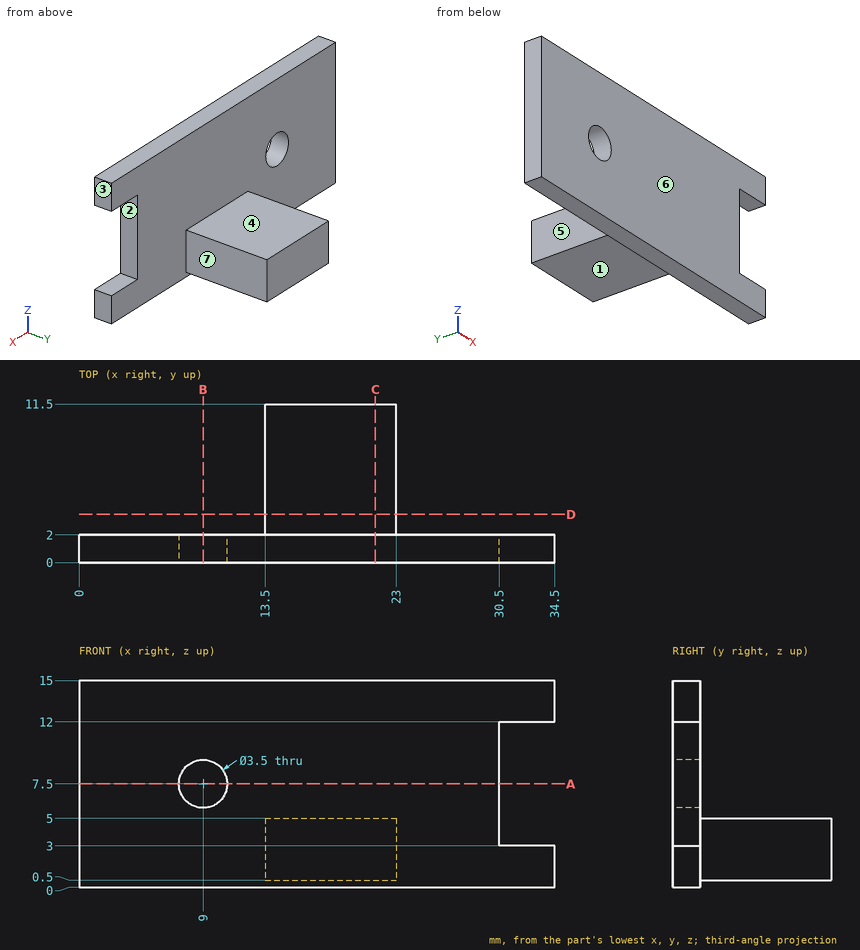
Geometry check sheet. Reference: drawing and pictorial views, mm from the part's lowest x, y, z. A direction names the side the tool comes from. Give positions to 0.01 mm unless a question says otherwise; leave off trailing zeros. Order: outer loops, then holes, each group sorted by start corner. A loop starts at its lowest first (then second) coordinate and runs counter-clockwise, first axis right, second up. Notation, with made-up numbers: M 36.25,1 L 43.25,1 A5 cw 43.25,5 Z; hole C 30.25,-10.5 d4. An arc over 180 degrees is marked long. Return JSON: item names as keys, results as strings. Group by question number.
1) Section check D-D on y = 3.5. Record the cut outline in (x, z).
2) Access from +Z, -Z, +X, -X, +Y, -Y to the whole of each face (thin tool, end or side, straight path). Record for the marked faces 4, 5, 6 and 7.
3) Go/stop test with flat-tipped pins: pin 1 Ø6 at (y, z) = (9.5, 5.5) entering from +X; pin 2 Ø5 at (y, z) = (5.5, 4) entering from -X; pin 3 Ø4.5 at (x, z) = (26, 8.5) entering from +Y. Record where each tip stops, or that it passes through.
4) Section check C-C on x = 21.5. Record the cut outline in (y, z), and give its area (4 significant figures).
5) Mould release check, pull along Z, two halves, no side actions. Record for the marked faces 1, 2 and 3: pulls with the +Z half, pulls with the -Z half, needs draft (parallel to the pull), parting line crosses it, or undercut.
6) Scan lines: line 1 (X direction, y = 0.4, z = 7.5); line 2 (Z direction, x = 9, y = 1.1); line 3 (Z direction, x = 15.5, y = 2.25). Record each from-to range of solid material in increasing order.
7) Section check B-B on x = 9. Record the cut outline in (y, z).
8) Section check A-A on z = 7.5. Record the cut outline in (x, y), and give its area (3 significant figures).
Answer block:
{
 "1": {"outline": "M 13.5,0.5 L 23,0.5 L 23,5 L 13.5,5 Z"},
 "2": {"face 4": "+Z, +X, -X, +Y", "face 5": "+Z, -Z, -X, +Y", "face 6": "+Z, -Z, +X, -X, -Y", "face 7": "+Z, -Z, +X, +Y"},
 "3": {"pin 1": "stops at x = 23", "pin 2": "stops at x = 13.5", "pin 3": "stops at y = 2"},
 "4": {"outline": "M 0,0 L 2,0 L 2,0.5 L 11.5,0.5 L 11.5,5 L 2,5 L 2,15 L 0,15 Z", "area": "72.75 mm^2"},
 "5": {"face 1": "pulls with the -Z half", "face 2": "undercut", "face 3": "needs draft"},
 "6": {"line 1": "x = 0 to 7.25, 10.75 to 30.5", "line 2": "z = 0 to 5.75, 9.25 to 15", "line 3": "z = 0.5 to 5"},
 "7": {"outline": "M 0,0 L 2,0 L 2,5.75 L 0,5.75 Z; M 0,9.25 L 2,9.25 L 2,15 L 0,15 Z"},
 "8": {"outline": "M 0,0 L 7.25,0 L 7.25,2 L 0,2 Z; M 10.75,0 L 30.5,0 L 30.5,2 L 10.75,2 Z", "area": "54.0 mm^2"}
}
